The listing builds one solid part. Answer for the finished solid, in the listing's coordinates (mm). A direction names the side the tool comes from. Give positions to 0.01 mm unless a question says otherwise; leave off trailing zeros. Answer in a Markdown table with one row per item. Add a question column.
from build123d import *

# Parameters (mm, degrees)
BOSS_EXTRUDE1_START = -2
BOSS_EXTRUDE1_DEPTH = 2
CUT_EXTRUDE1_REACH  = 34.718
SKETCH2_3_R         = 2.25
FILLET1_R           = 7.3
FILLET2_R           = 2.7
CHAMFER1_SIZE       = 1.154700538
CHAMFER1_SIZE_2     = 2
CHAMFER2_SIZE       = 3
FILLET3_R           = 5
CHAMFER3_SIZE       = 2


with BuildPart() as part:
    # Sketch1 → Revolve1 (revolve)
    with BuildSketch(Plane.XY, mode=Mode.PRIVATE) as revolve1_sk:
        Polygon((-5, 0), (-5, 2), (-18.6, 2), (-18.6, 0), (-10.25, 0), (-10.25, -6), (-5, -6), align=None)
    revolve(revolve1_sk.sketch.rotate(Axis((0, 9.858601723, 0), (0, -1, 0)), 270), axis=Axis((0, 9.858601723, 0), (0, -1, 0)))

    # Sketch2 → Boss-Extrude1 (add)
    with BuildSketch(Plane(origin=(0, 2, 0), x_dir=(1, 0, 0), z_dir=(0, 1, 0)).offset(BOSS_EXTRUDE1_START)):
        with BuildLine():
            Line((-5.7, 25.7), (-5.7, 17.705084016))
            ThreePointArc((-5.7, 17.705084016), (-3.720937263, 18.224012343), (-1.696852692, 18.5224375))
            ThreePointArc((-1.696852692, 18.5224375), (-0.788854056, 22.10718041), (2.25, 20))
            ThreePointArc((2.25, 20), (2.10718041, 19.211145944), (1.696852692, 18.5224375))
            ThreePointArc((1.696852692, 18.5224375), (3.720937263, 18.224012343), (5.7, 17.705084016))
            Line((5.7, 17.705084016), (5.7, 25.7))
            Line((5.7, 25.7), (0.005376723, 25.7))
            Line((0.005376723, 25.7), (-0.005376723, 25.7))
            Line((-0.005376723, 25.7), (-5.7, 25.7))
        make_face()
        with BuildLine():
            ThreePointArc((-1.696852692, -18.5224375), (-3.720937263, -18.224012343), (-5.7, -17.705084016))
            Line((-5.7, -17.705084016), (-5.7, -25.7))
            Line((-5.7, -25.7), (-0.005376723, -25.7))
            Line((-0.005376723, -25.7), (0.005376723, -25.7))
            Line((0.005376723, -25.7), (5.7, -25.7))
            Line((5.7, -25.7), (5.7, -17.705084016))
            ThreePointArc((5.7, -17.705084016), (3.720937263, -18.224012343), (1.696852692, -18.5224375))
            ThreePointArc((1.696852692, -18.5224375), (2.10718041, -19.211145944), (2.25, -20))
            ThreePointArc((2.25, -20), (-0.788854056, -22.10718041), (-1.696852692, -18.5224375))
        make_face()
    extrude(amount=BOSS_EXTRUDE1_DEPTH)

    # Sketch2<3> → Cut-Extrude1 (cut, up to next)
    with BuildSketch(Plane(origin=(0, 2, 0), x_dir=(1, 0, 0), z_dir=(0, 1, 0)), mode=Mode.PRIVATE) as cut_extrude1_sk1:
        with Locations(Location((0, 20, 0), (0, 0, 270))):
            Circle(SKETCH2_3_R)
    cut_extrude1_tool1 = extrude(cut_extrude1_sk1.sketch, amount=-CUT_EXTRUDE1_REACH, mode=Mode.PRIVATE) & part.part
    # Sketch2<3> → Cut-Extrude1 (cut, up to next)
    with BuildSketch(Plane(origin=(0, 2, 0), x_dir=(1, 0, 0), z_dir=(0, 1, 0)), mode=Mode.PRIVATE) as cut_extrude1_sk2:
        with Locations(Location((0, -20, 0), (0, 0, 270))):
            Circle(SKETCH2_3_R)
    cut_extrude1_tool2 = extrude(cut_extrude1_sk2.sketch, amount=-CUT_EXTRUDE1_REACH, mode=Mode.PRIVATE) & part.part
    add(cut_extrude1_tool1.solids().sort_by_distance((0, 2, -20))[0], mode=Mode.SUBTRACT)
    add(cut_extrude1_tool2.solids().sort_by_distance((0, 2, 20))[0], mode=Mode.SUBTRACT)

    # Fillet1
    fillet1_edges = [part.edges().sort_by_distance(p)[0] for p in [
        (-5.7, 1, -17.705084016),
        (5.7, 1, -17.705084016),
        (-5.7, 1, 17.705084016),
        (5.7, 1, 17.705084016),
    ]]
    fillet(fillet1_edges, radius=FILLET1_R)

    # Fillet2
    fillet2_edges = [part.edges().sort_by_distance(p)[0] for p in [
        (-5.7, 1, -25.7),
        (5.7, 1, -25.7),
        (-5.7, 1, 25.7),
        (5.7, 1, 25.7),
    ]]
    fillet(fillet2_edges, radius=FILLET2_R)

    # Chamfer1
    # the kernel refuses this chamfer: 2, 1.154700538 mm, written as the material it takes off along each edge
    with BuildSketch(Plane(origin=(3, 2, 25.7), x_dir=(0, 0.05789386240267148, -0.9983227437537925), z_dir=(-1, 0, 0)), Plane(origin=(-3, 2, -25.7), x_dir=(0, 0.05789386240267148, 0.9983227437537925), z_dir=(1, 0, 0))) as chamfer1_piece_1:
        Polygon((CHAMFER1_SIZE * 0.998322744082, CHAMFER1_SIZE * 0.0578938624217), (-CHAMFER1_SIZE_2 * 0.0578938624027, CHAMFER1_SIZE_2 * 0.998322743754), (0, 0), align=None)
    extrude(amount=6, mode=Mode.SUBTRACT)
    with BuildSketch(Plane(origin=(5.7, 2, 23), x_dir=(-0.9983227437537925, 0.05789386240267148, 0), z_dir=(0, 0, -1)), Plane(origin=(-5.7, 2, 22.401116044), x_dir=(0.9983227437537925, 0.05789386240267148, 0), z_dir=(0, 0, 1)), Plane(origin=(5.7, 2, -22.401116044), x_dir=(-0.9983227437537925, 0.05789386240267148, 0), z_dir=(0, 0, -1)), Plane(origin=(-5.7, 2, -23), x_dir=(0.9983227437537925, 0.05789386240267148, 0), z_dir=(0, 0, 1))) as chamfer1_piece_2:
        Polygon((CHAMFER1_SIZE * 0.998322744082, -CHAMFER1_SIZE * 0.0578938624217), (-CHAMFER1_SIZE_2 * 0.0578938624027, -CHAMFER1_SIZE_2 * 0.998322743754), (0, 0), align=None)
    extrude(amount=0.598883956, mode=Mode.SUBTRACT)
    with BuildSketch(Plane(origin=(13, 2, 22.401116044), x_dir=(-1, 0, 0), z_dir=(0, 0, 1))) as chamfer1_piece_3:
        Polygon((7.3 + CHAMFER1_SIZE, 0), (7.3, CHAMFER1_SIZE_2), (7.3, 0), align=None)
    revolve(axis=Axis((13, 2, 22.401116044), (0, -1, 0)), revolution_arc=59.87219662, mode=Mode.SUBTRACT)
    with BuildSketch(Plane(origin=(-13, 2, 22.401116044), x_dir=(0.5019305019305016, 0, -0.8649079553523569), z_dir=(-0.8649079553523569, 0, -0.5019305019305016))) as chamfer1_piece_4:
        Polygon((7.3 + CHAMFER1_SIZE, 0), (7.3, CHAMFER1_SIZE_2), (7.3, 0), align=None)
    revolve(axis=Axis((-13, 2, 22.401116044), (0, -1, 0)), revolution_arc=59.87219662, mode=Mode.SUBTRACT)
    with BuildSketch(Plane(origin=(0, 2, 0), x_dir=(0.5019305019305017, 0, -0.8649079553523569), z_dir=(-0.8649079553523569, 0, -0.5019305019305017))) as chamfer1_piece_5:
        Polygon((18.6 - CHAMFER1_SIZE, 0), (18.6, CHAMFER1_SIZE_2), (18.6, 0), align=None)
    revolve(axis=Axis((0, 2, 0), (0, -1, 0)), revolution_arc=119.74439324, mode=Mode.SUBTRACT)
    with BuildSketch(Plane(origin=(0, 2, 0), x_dir=(-0.5019305019305019, 0, 0.8649079553523568), z_dir=(0.8649079553523568, 0, 0.5019305019305019))) as chamfer1_piece_6:
        Polygon((18.6 - CHAMFER1_SIZE, 0), (18.6, CHAMFER1_SIZE_2), (18.6, 0), align=None)
    revolve(axis=Axis((0, 2, 0), (0, -1, 0)), revolution_arc=119.74439324, mode=Mode.SUBTRACT)
    with BuildSketch(Plane(origin=(13, 2, -22.401116044), x_dir=(-1, 0, 0), z_dir=(0, 0, -1))) as chamfer1_piece_7:
        Polygon((7.3 + CHAMFER1_SIZE, 0), (7.3, -CHAMFER1_SIZE_2), (7.3, 0), align=None)
    revolve(axis=Axis((13, 2, -22.401116044), (0, 1, 0)), revolution_arc=59.87219662, mode=Mode.SUBTRACT)
    with BuildSketch(Plane(origin=(-13, 2, -22.401116044), x_dir=(0.5019305019305013, 0, 0.8649079553523572), z_dir=(-0.8649079553523572, 0, 0.5019305019305013))) as chamfer1_piece_8:
        Polygon((7.3 + CHAMFER1_SIZE, 0), (7.3, -CHAMFER1_SIZE_2), (7.3, 0), align=None)
    revolve(axis=Axis((-13, 2, -22.401116044), (0, 1, 0)), revolution_arc=59.87219662, mode=Mode.SUBTRACT)
    with BuildSketch(Plane(origin=(3, 2, 23), x_dir=(0, 0, 1), z_dir=(-1, 0, 0))) as chamfer1_piece_9:
        Polygon((2.7 - CHAMFER1_SIZE, 0), (2.7, -CHAMFER1_SIZE_2), (2.7, 0), align=None)
    revolve(axis=Axis((3, 2, 23), (0, 1, 0)), revolution_arc=90, mode=Mode.SUBTRACT)
    with BuildSketch(Plane(origin=(-3, 2, 23), x_dir=(-1, 0, 0), z_dir=(0, 0, -1))) as chamfer1_piece_10:
        Polygon((2.7 - CHAMFER1_SIZE, 0), (2.7, -CHAMFER1_SIZE_2), (2.7, 0), align=None)
    revolve(axis=Axis((-3, 2, 23), (0, 1, 0)), revolution_arc=90, mode=Mode.SUBTRACT)
    with BuildSketch(Plane(origin=(3, 2, -23), x_dir=(0, 0, -1), z_dir=(-1, 0, 0))) as chamfer1_piece_11:
        Polygon((2.7 - CHAMFER1_SIZE, 0), (2.7, CHAMFER1_SIZE_2), (2.7, 0), align=None)
    revolve(axis=Axis((3, 2, -23), (0, -1, 0)), revolution_arc=90, mode=Mode.SUBTRACT)
    with BuildSketch(Plane(origin=(-3, 2, -23), x_dir=(-1, 0, 0), z_dir=(0, 0, 1))) as chamfer1_piece_12:
        Polygon((2.7 - CHAMFER1_SIZE, 0), (2.7, CHAMFER1_SIZE_2), (2.7, 0), align=None)
    revolve(axis=Axis((-3, 2, -23), (0, -1, 0)), revolution_arc=90, mode=Mode.SUBTRACT)

    # Chamfer2
    chamfer2_edges = [part.edges().sort_by_distance(p)[0] for p in [
        (0, 2, -5),
    ]]
    chamfer(chamfer2_edges, length=CHAMFER2_SIZE)

    # Fillet3
    fillet3_edges = [part.edges().sort_by_distance(p)[0] for p in [
        (0, -1, -5),
    ]]
    fillet(fillet3_edges, radius=FILLET3_R)

    # Chamfer3
    chamfer3_edges = [part.edges().sort_by_distance(p)[0] for p in [
        (0, 0, -10.25),
    ]]
    chamfer(chamfer3_edges, length=CHAMFER3_SIZE)


solid = part.part
1. Given pin 1 Ø8 at (x, z) = (0, 0) entering from -Y; pin 2 Ø12 at (x, z) = (-4, 4) entering from +Y; pin 3 Ø4 at (x, y) = (5, -2.5) entering from +Z, each flat-ended and moving along its own axis, determine where each tip first touches the part or whether it passes through.
2. Section A-A (x = 0) is taken. State how many separate pieces and enclosed holes the cut face has, and give its area (3 significant figures).
3. A tool of negligible diameter and unlimited length cuts with its end or side. For faces 4 (the face through (-5.115, 1.014, -22.705)), 5 (the face through (5.115, 1.014, 22.705)), 6 (the face through (10.006, -4.028, -2.222)), from which of +Z, -Z, +X, -X, +Y, -Y can it reach the whole face along a straight path? Write none if from no direction.
4. Straight lines are drawn through the part: L1, parallel to X at y = -4, z = 0; L2, parallel to Y at x = 11.5, z = 13; L3, parallel to X at y = -1, z = 4. For each, find the intervals that lie inside material, in ascending order. Write a range as [from, to].
5. The mould has two halves that part along X. Classify faces 1 (the face through (-8, 2, 6)), 2 (the face through (-1.5, -4.52, 4.77)), 3 (the face through (5.115, 1.014, -22.696)): +X half, -X half, draft (parallel to the pull), parting line (faces both ways), or undercut.
Geometry check:
| question | item | result |
|---|---|---|
| 1 | pin 1 | through |
| 1 | pin 2 | y = 2 |
| 1 | pin 3 | z = 10.8 |
| 2 | separate pieces | 4 |
| 2 | enclosed holes | 0 |
| 2 | area | 119 mm² |
| 3 | face 4 | -Z, -X, +Y |
| 3 | face 5 | +Z, +X, +Y |
| 3 | face 6 | -Y |
| 4 | L1 | [-10.25, -5], [5, 10.25] |
| 4 | L2 | [0, 2] |
| 4 | L3 | [-10.51, -3.7], [3.7, 10.51] |
| 5 | face 1 | draft |
| 5 | face 2 | undercut |
| 5 | face 3 | +X half |
